For this review, use the dimensioned drawing (mm, ordinates from the lowest corner) and the shaded views. Coordinates: 2 decimals unless noted, no trailing zeros. Write each loop counter-clockwise with the first axis right and the second up, starting at its lowest first coordinate (ties: lowest second). Pieces come first, ordered by that corner, then holes. Notation, with made-up numbers: (-4, -26.75) - (47, -26.75) arc R37 ccw to (47, 11.25) - close; hole circle Ø11 at (52.5, 1). An arc over 180 degrees is marked (long way). One line per item, written item: value.
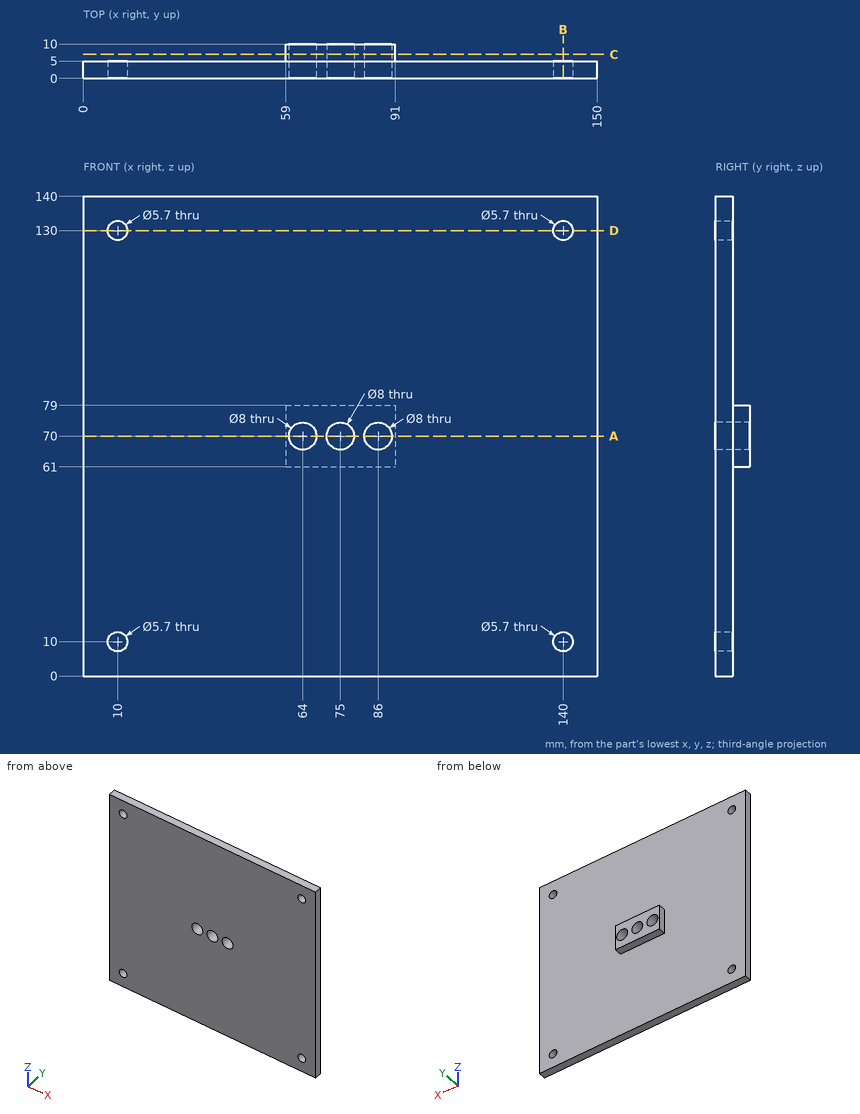
1. Consider section A-A, the plane z = 70. Write out the cut boundary in (x, y).
Answer block:
outline: (0, 0) - (60, 0) - (60, 10) - (59, 10) - (59, 5) - (0, 5) - close; (68, 0) - (71, 0) - (71, 10) - (68, 10) - close; (79, 0) - (82, 0) - (82, 10) - (79, 10) - close; (90, 0) - (150, 0) - (150, 5) - (91, 5) - (91, 10) - (90, 10) - close
2. Consider section C-C, the plane y = 7. Write out the cut boundary in (x, z).
Answer block:
outline: (59, 61) - (91, 61) - (91, 79) - (59, 79) - close; hole circle Ø8 at (64, 70); hole circle Ø8 at (75, 70); hole circle Ø8 at (86, 70)
3. Wall thickness on line 1 along Z through (x, y) = (140, 1.8); line 2 along X through (y, z) = (3.4, 130); line 3 along X through (y, z) = (6.75, 70): over which ranges is each line inside the solid? List them lowest first.
Answer block:
line 1: z = 0 to 7.15, 12.85 to 127.15, 132.85 to 140
line 2: x = 0 to 7.15, 12.85 to 137.15, 142.85 to 150
line 3: x = 59 to 60, 68 to 71, 79 to 82, 90 to 91
4. Consider section D-D, the plane z = 130. Write out the cut boundary in (x, y), then the cut area to 3 significant figures.
Answer block:
outline: (0, 0) - (7.15, 0) - (7.15, 5) - (0, 5) - close; (12.85, 0) - (137.15, 0) - (137.15, 5) - (12.85, 5) - close; (142.85, 0) - (150, 0) - (150, 5) - (142.85, 5) - close
area: 693 mm^2
5. Insertion check: pin 1 Ø4.5 at (x, z) = (10, 10) entering from +Y; pin 2 Ø6.5 at (x, z) = (10, 130) entering from +Y; pin 3 Ø2.5 at (x, y) = (79, 6.5) entering from -Z; pin 4 Ø2.5 at (y, z) = (6.5, 71) entering from +X. Each pin has a flat end and moves straight along its axis. Give the tip position at first contact, or say it passes through.
Answer block:
pin 1: passes through
pin 2: stops at y = 5
pin 3: stops at z = 61
pin 4: stops at x = 91
6. Consider section B-B, the plane x = 140. Write out the cut boundary in (y, z).
Answer block:
outline: (0, 0) - (5, 0) - (5, 7.15) - (0, 7.15) - close; (0, 12.85) - (5, 12.85) - (5, 127.15) - (0, 127.15) - close; (0, 132.85) - (5, 132.85) - (5, 140) - (0, 140) - close
